Design review of the part shown in the three views and the two pictorial views. Dimensions are in mm from the part's minimum x, y and z. Give positions to 0.01 mm unless a question says otherwise; leave off trailing zeros. Order: outer loops, then holes, each group sorted by start corner. A loop starts at its lowest first (then second) coordinate and runs counter-clockwise, first axis right, second up. Notation, with made-up numbers: M -38.75,30 L 2.25,30 A13 ccw 2.25,50 Z; hole C 6.25,86 d1. An arc over 180 degrees is marked long. Answer as a JSON object with one key per item and string values.
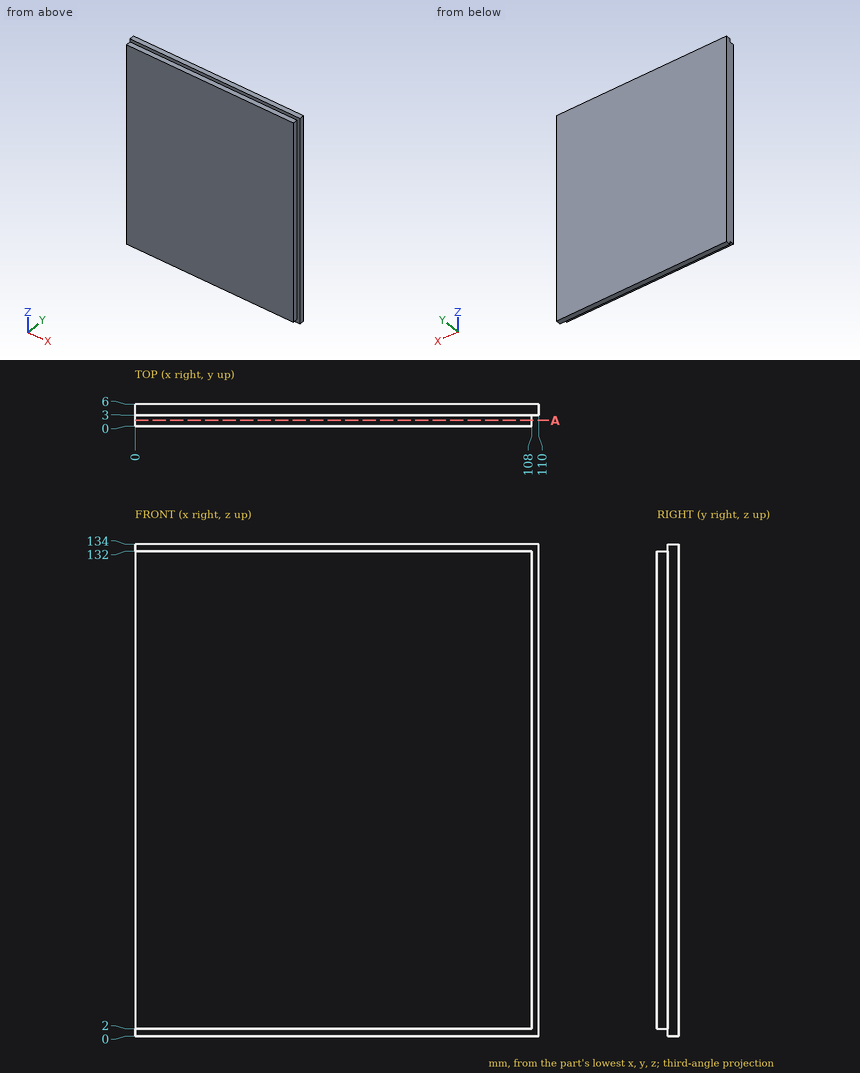
(1) We need section A-A (y = 1.55). Write out the cut boundary in (x, z).
Checked values:
{"outline": "M 0,2 L 108,2 L 108,132 L 0,132 Z"}
(2) Insertion check: pin 1 (1.5 mm diameter, centred on x = 29.5, y = 2, fed in from +Z); pin 2 (0.9 mm diameter, centred on x = 76.5, y = 1.5, fed in from -Z); pin 3 (2.5 mm diameter, centred on y = 1, z = 62.5, fed in from +X). Each pin has a flat end and moves straight along its axis. Give the tip position at first contact, or say it passes through.
Checked values:
{"pin 1": "stops at z = 132", "pin 2": "stops at z = 2", "pin 3": "stops at x = 108"}
(3) To check wall thickness, follow L1, parallel to X at y = 0.5, z = 58; L2, parallel to Z at x = 96, y = 0.65. State the ranges of each line that lie inside material, in increasing order. Write a range as from..to.
Checked values:
{"L1": "x = 0..108", "L2": "z = 2..132"}
